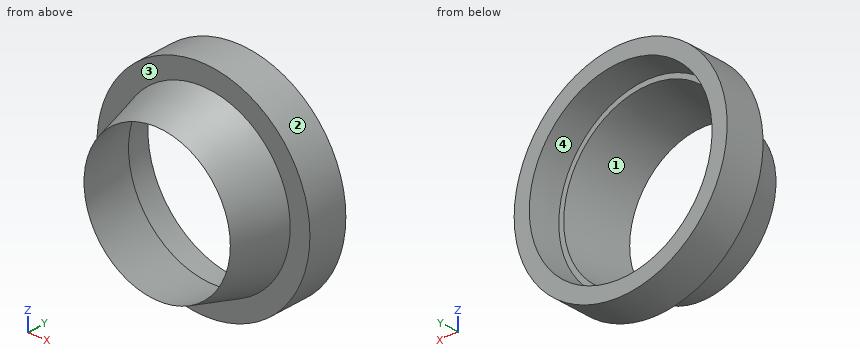
Solid Edge part; units mm, degrees
sketch "Sketch1" plane through (0, 0, 0) normal (0, 0, 1) x (1, 0, 0)
  line L0 (43.184, 24) -> (35.184, 24)
  line L1 (35.184, 24) -> (29.6588, 3.3798)
  line L2 (29.6588, 3.3798) -> (34, 28)
  line L3 (34, 28) -> (36, 28)
  line L4 (36, 28) -> (37.0499, 40)
  line L5 (37.0499, 40) -> (43.184, 40)
  line L6 (43.184, 40) -> (43.184, 24)
revolve "RevolvedProtrusion1" add sketch "Sketch1" angle 360 about axis through (0, 0, 0) along (0, 1, 0)
properties material "Policarbonato"
Can you work these out from the model? Positions are in its coordinate system, mm. Face numbers are marked on the shaded views. Give positions to 0.01 mm unless a question says otherwise; leave off trailing zeros. Loops run counter-clockwise (first coordinate to the right, second up) from the corner with the lowest first, then second, coordinate; pieces in that order, holes last. Notation, with made-up numbers: (79.5, 24) -> (135.5, 24) arc R31 cw to (135.5, 51) -> close; hole circle Ø4 at (4, 1.5). An arc over 180 degrees is marked (long way). Return JSON: item names as keys, results as strings.
Q1. I need wall thicknesses on probe 1 along Y at (x, z) = (-34.5, 21); probe 2 along Z at (x, y) = (-25, 30.5); probe 3 along X at (y, z) = (19, -27.5). Which ranges of each line are inside material? Lowest first, please.
Checks:
{"probe 1": "y = 24 to 40", "probe 2": "z = -35.21 to -26.21, 26.21 to 35.21", "probe 3": "x = -19.73 to -17.16, 17.16 to 19.73"}
Q2. I want a section at C-C, the plane y = 37. List the corners of the cut face in (x, z) for me, then the cut area to 3 significant figures.
Checks:
{"outline": "circle Ø86.37 at (0, 0); hole circle Ø73.57 at (0, 0)", "area": "1,610 mm2"}
Q3. I want a section at A-A, the plane z = 0. List the corners of the cut face in (x, y) for me, then the cut area to 3 significant figures.
Checks:
{"outline": "(-43.18, 24) -> (-35.18, 24) -> (-29.66, 3.38) -> (-34, 28) -> (-36, 28) -> (-37.05, 40) -> (-43.18, 40) -> close; (29.66, 3.38) -> (35.18, 24) -> (43.18, 24) -> (43.18, 40) -> (37.05, 40) -> (36, 28) -> (34, 28) -> close", "area": "275 mm2"}
Q4. I want a section at D-D, the plane y = 12.5. List the corners of the cut face in (x, z) for me, then the cut area to 3 significant figures.
Checks:
{"outline": "circle Ø64.21 at (0, 0); hole circle Ø62.53 at (0, 0)", "area": "166 mm2"}
Q5. We'd pull the mould along X, two halves only. Please class the marked faces 1, 2, 3 and 4: released by +X, released by -X, zero draft, split by the parting line, or undercut.
Checks:
{"face 1": "undercut", "face 2": "split by the parting line", "face 3": "zero draft", "face 4": "undercut"}
Q6. For pin 1 Ø1.5 at (x, z) = (25.5, -23.5) entering from +Y; pin 2 Ø1 at (x, y) = (-4, 26) entering from +Z; pin 3 Ø5 at (x, y) = (-28.5, 27) entering from -Z; pin 4 Ø8 at (x, z) = (-14.5, 18) entering from -Y, each with a flat end and sliding along its axis, tell me the tip position at first contact or that it passes through.
Checks:
{"pin 1": "stops at y = 28", "pin 2": "stops at z = 43.04", "pin 3": "stops at z = -34.48", "pin 4": "passes through"}
Q7. I want a section at B-B, the plane x = 0. List the corners of the cut face in (y, z) for me, then the cut area to 3 significant figures.
Checks:
{"outline": "(3.38, -29.66) -> (24, -35.18) -> (24, -43.18) -> (40, -43.18) -> (40, -37.05) -> (28, -36) -> (28, -34) -> close; (3.38, 29.66) -> (28, 34) -> (28, 36) -> (40, 37.05) -> (40, 43.18) -> (24, 43.18) -> (24, 35.18) -> close", "area": "275 mm2"}
